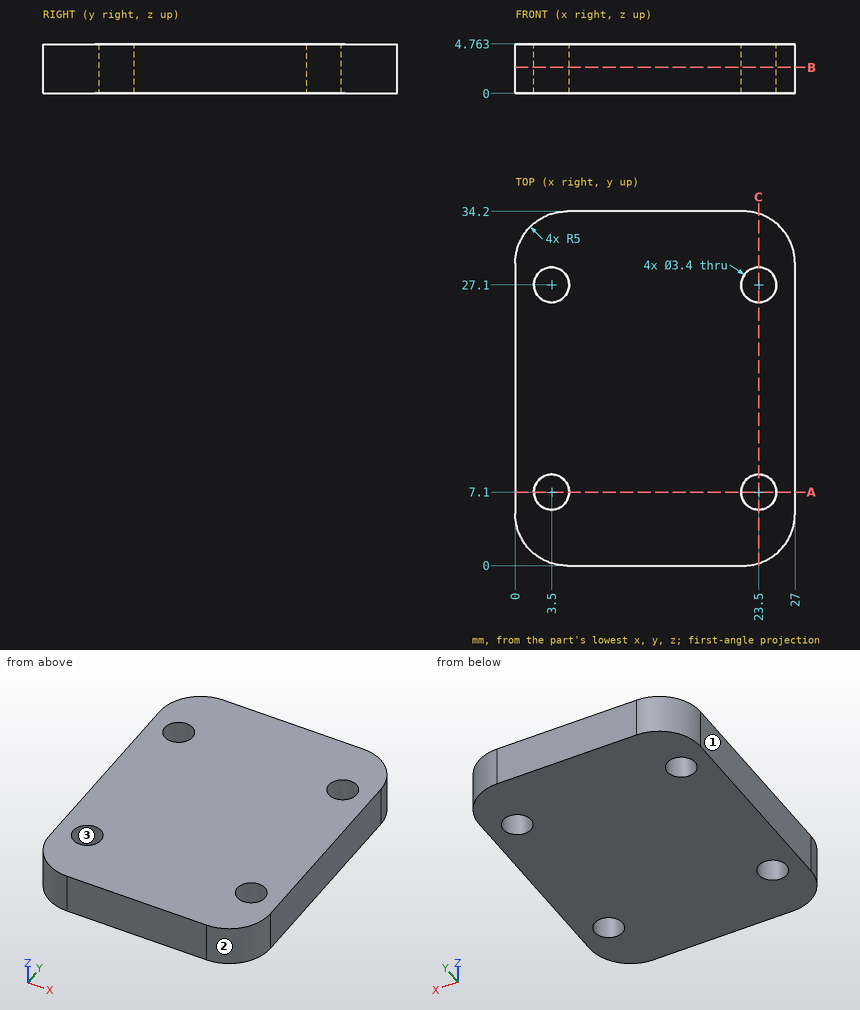
The drawing under review shows one solid part. Ordinate dimensions are in mm from its lowest x, y, z. Coordinates: 2 decimals unless noted, no trailing zeros. Loops run counter-clockwise (first coordinate to the right, second up) from the corner with the lowest first, then second, coordinate; pieces in that order, holes last. Notation, with made-up numbers: M 35.25,-35.5 L 86.25,-35.5 A20 ccw 86.25,1.5 Z; hole C -2,-37.75 d10. An arc over 180 degrees is marked long. Use one line per item in the form item = value.
(1) Consider section C-C (x = 23.5). Write out the cut boundary in (y, z).
Return value:
outline = M 0.23,0 L 5.4,0 L 5.4,4.76 L 0.23,4.76 Z; M 8.8,0 L 25.4,0 L 25.4,4.76 L 8.8,4.76 Z; M 28.8,0 L 33.97,0 L 33.97,4.76 L 28.8,4.76 Z
(2) For line 1 along X through (y, z) = (27.1, 2.1); line 2 along X through (y, z) = (6, 0.6) (1 decimal); line 3 along Y through (x, z) = (23.5, 1.5), list the stretches that pass through material, from the lowest coordinate up. Write a range as from..to.
Return value:
line_1 = 0..1.8, 5.2..21.8, 25.2..27
line_2 = 0..2.2, 4.8..22.2, 24.8..27
line_3 = 0.23..5.4, 8.8..25.4, 28.8..33.97
(3) Clearance check with flat-ended pins moving along their axes: P1, Ø8, axis at x = 21.5, y = 16, coming from the -Z side; P2, Ø2, axis at x = 23.5, y = 7.1, coming from the +Z side (3 decimals). State where each tip first meets the part, or that it passes through.
Return value:
P1 = 0
P2 = through
(4) Consider section A-A (y = 7.1). Write out the cut boundary in (x, z).
Return value:
outline = M 0,0 L 1.8,0 L 1.8,4.76 L 0,4.76 Z; M 5.2,0 L 21.8,0 L 21.8,4.76 L 5.2,4.76 Z; M 25.2,0 L 27,0 L 27,4.76 L 25.2,4.76 Z
(5) Consider section B-B (z = 2.5). Write out the cut boundary in (x, y).
Return value:
outline = M 0,5 A5 ccw 5,0 L 22,0 A5 ccw 27,5 L 27,29.2 A5 ccw 22,34.2 L 5,34.2 A5 ccw 0,29.2 Z; hole C 3.5,7.1 d3.4; hole C 3.5,27.1 d3.4; hole C 23.5,7.1 d3.4; hole C 23.5,27.1 d3.4
(6) Draft analysis for pull direction Y (two halves, no side actions). For the marked faces 1, 2 and 3, state which applies: pulls with the +Y half, pulls with the -Y half, needs draft (parallel to the pull), parting line crosses it, or undercut.
Return value:
face_1 = needs draft
face_2 = pulls with the -Y half
face_3 = undercut
